```python
from build123d import *

# Parameters (mm, degrees)
BOSS_EXTRUDE1_DEPTH      = 7.5
BOSS_EXTRUDE2_DEPTH      = 18.54
BOSS_EXTRUDE2_DEPTH_BACK = 22.877829
CUT_EXTRUDE2_START       = -22.877828503
CUT_EXTRUDE2_DEPTH       = 22.877828503
CUT_EXTRUDE1_DEPTH       = 7.5


with BuildPart() as part:
    # Sketch2 → Boss-Extrude1 (new body)
    with BuildSketch(Plane.XY):
        with BuildLine():
            Line((75.649019024, 29.060438862), (108.081997982, 29.060438862))
            Line((108.081997982, 29.060438862), (108.081997982, 6.182610359))
            Line((108.081997982, 6.182610359), (12.081997982, 6.182610359))
            Line((12.081997982, 6.182610359), (12.081997982, 29.060438862))
            Line((12.081997982, 29.060438862), (47.250085178, 29.060438862))
            Line((47.250085178, 29.060438862), (47.250085178, 24.305651432))
            ThreePointArc((47.250085178, 24.305651432), (61.326511028, 9.983143436), (75.649019024, 24.059569287))
            Line((75.649019024, 24.059569287), (75.649019024, 29.060438862))
        make_face()
    extrude(amount=BOSS_EXTRUDE1_DEPTH)

    # Sketch7 → Boss-Extrude2 (add, two sides: drawn at the far end of the back side and taken through both)
    with BuildSketch(Plane(origin=(0, 29.060438862, 0), x_dir=(1, 0, 0), z_dir=(0, 1, 0)).offset(-BOSS_EXTRUDE2_DEPTH_BACK)):
        with BuildLine():
            Line((101.320347636, 0), (103.631986296, 0))
            ThreePointArc((103.631986296, 0), (105.511041931, -3.678722762), (107.080019787, -7.5))
            Line((107.080019787, -7.5), (104.946394262, -7.5))
            ThreePointArc((104.946394262, -7.5), (103.296384641, -3.6711873), (101.320347636, 0))
        make_face()
        with BuildLine():
            Line((18.843648328, 0), (16.532009668, 0))
            ThreePointArc((16.532009668, 0), (14.652954033, -3.678722762), (13.083976177, -7.5))
            Line((13.083976177, -7.5), (15.217601702, -7.5))
            ThreePointArc((15.217601702, -7.5), (16.867611323, -3.6711873), (18.843648328, 0))
        make_face()
    extrude(amount=BOSS_EXTRUDE2_DEPTH + BOSS_EXTRUDE2_DEPTH_BACK)

    # Sketch9 → Cut-Extrude2 (cut)
    with BuildSketch(Plane(origin=(0, 29.060438862, 0), x_dir=(1, 0, 0), z_dir=(0, 1, 0)).offset(CUT_EXTRUDE2_START)):
        with BuildLine():
            Line((108.081997982, 0), (103.631986296, 0))
            ThreePointArc((103.631986296, 0), (105.511041931, -3.678722762), (107.080019787, -7.5))
            Line((107.080019787, -7.5), (108.081997982, -7.5))
            Line((108.081997982, -7.5), (108.081997982, 0))
        make_face()
        with BuildLine():
            Line((12.081997982, -7.5), (13.083976177, -7.5))
            ThreePointArc((13.083976177, -7.5), (14.652954033, -3.678722762), (16.532009668, 0))
            Line((16.532009668, 0), (12.081997982, 0))
            Line((12.081997982, 0), (12.081997982, -7.5))
        make_face()
    extrude(amount=CUT_EXTRUDE2_DEPTH, mode=Mode.SUBTRACT)

    # Sketch8 → Cut-Extrude1 (cut)
    with BuildSketch(Plane.XY.offset(7.5)):
        with BuildLine():
            Line((18.843648328, 25.060438862), (18.843648328, 9.983143436))
            Line((18.843648328, 9.983143436), (50.064839288, 9.983143436))
            add(Edge.make_bspline(
                [(50.064839288, 9.983143436), (45.21005588, 13.875585407), (43.215886983, 19.247270307), (43.250085178, 24.305651432)],
                knots=[0.673696083, 0.673696083, 0.673696083, 0.673696083, 1, 1, 1, 1], degree=3, weights=[0.560759297, 0.636257623, 0.782671191, 1]))
            Line((43.250085178, 24.305651432), (43.250085178, 25.060438862))
            Line((43.250085178, 25.060438862), (18.843648328, 25.060438862))
        make_face()
        with BuildLine():
            Line((101.320347636, 9.983143436), (101.320347636, 25.060438862))
            Line((101.320347636, 25.060438862), (79.649019024, 25.060438862))
            Line((79.649019024, 25.060438862), (79.648868861, 24.02490983))
            add(Edge.make_bspline(
                [(79.648868861, 24.02490983), (79.605779212, 19.052181459), (77.595427824, 13.800428938), (72.83438207, 9.983143436)],
                knots=[0, 0, 0, 0, 0.321967204, 0.321967204, 0.321967204, 0.321967204], degree=3, weights=[1, 0.78555958, 0.640161942, 0.563807087]))
            Line((72.83438207, 9.983143436), (101.320347636, 9.983143436))
        make_face()
    extrude(amount=-CUT_EXTRUDE1_DEPTH, mode=Mode.SUBTRACT)


solid = part.part
```
Source: CAD feature listing. Evaluate the final solid. Frame: model axes, mm. A direction names the side the tool comes from. Round coordinates to 2 decimals unless told otherwise and drop trailing zeros. Loops run counter-clockwise (first coordinate to the right, second up) from the corner with the lowest first, then second, coordinate; pieces in that order, holes last.
1. Mould query, pull axis Y, two halves, no side actions, for faces 4 (the flat face through (101.32, 17, 4)), 5 (the flat face through (16, 47.6, 4)), 6 (the flat face through (75.649, 27, 4)). Classes: released by +Y, released by -Y, zero draft, split by the parting line, or undercut.
2. Section query C-C on z = 5.25. Give the number of separate pieces and of enclosed holes in the cut face, and give its area (3 significant figures).
3. Section query A-A on x = 23. Output: boundary loops of the cut face in (y, z).
4. Section query B-B on y = 35. Output: boundary loops of the cut face in (x, z).
5. Contact query for flat-ended pins moving along their axis: pin 1 (0.8 mm diameter, centred on y = 24.5, z = 5, fed in from -X); pin 2 (4 mm diameter, centred on x = 93, z = 5, fed in from +Y); pin 3 (1.5 mm diameter, centred on y = 34.5, z = 1.5, fed in from -X). Output: stop coordinate, or through.
6. Access query for faces 1 (the flat face through (47.25, 27, 4)), 2 (the cylindrical face through (16.842, 38.201, 3.724)), 3 (the flat face through (34, 9.983, 4)). Directions: +Z, -Z, +X, -X, +Y, -Y. A direction counts if a zero-diameter tool reaches every point of the face in a straight line with its end or side. Return the directions, or none.
7. Ray query, L1, parallel to Y at x = 82, z = 1.25; L2, parallel to X at y = 25.5, z = 2.5; L3, parallel to X at y = 20.5, z = 1.5. Return the intervals inside material, ascending.
Answers below:
1. face 4: undercut
1. face 5: released by +Y
1. face 6: zero draft
2. separate pieces: 1
2. enclosed holes: 2
2. area: 982 mm2
3. outline: (6.18, 0) - (9.98, 0) - (9.98, 7.5) - (6.18, 7.5) - close; (25.06, 0) - (29.06, 0) - (29.06, 7.5) - (25.06, 7.5) - close
4. outline: (13.08, 7.5) arc R50 ccw to (16.53, 0) - (18.84, 0) arc R48 cw to (15.22, 7.5) - close; (101.32, 0) - (103.63, 0) arc R50 ccw to (107.08, 7.5) - (104.95, 7.5) arc R48 cw to start
5. pin 1: stops at x = 13.9
5. pin 2: stops at y = 29.06
5. pin 3: stops at x = 15.34
6. face 1: +Z, -Z, +Y
6. face 2: +Z, +Y
6. face 3: +Z, -Z
7. L1: y = 6.18 to 9.98, 25.06 to 29.06
7. L2: x = 15.21 to 47.25, 75.65 to 104.95
7. L3: x = 15.72 to 18.84, 43.63 to 47.74, 75.16 to 79.27, 101.32 to 104.44
